from build123d import *

# Parameters (mm, degrees)
SKETCH1_R                                           = 18
BOSS_EXTRUDE1_DEPTH                                 = 7
CBORE_FOR_M4_HEX_SOCKET_HEAD_CAP_SCREW2_D           = 4.8
CBORE_FOR_M4_HEX_SOCKET_HEAD_CAP_SCREW2_DEPTH       = 10
CBORE_FOR_M4_HEX_SOCKET_HEAD_CAP_SCREW2_CBORE_D     = 8.2
CBORE_FOR_M4_HEX_SOCKET_HEAD_CAP_SCREW2_CBORE_DEPTH = 4.4
CBORE_FOR_M4_HEX_SOCKET_HEAD_CAP_SCREW2_TIP         = 1.442065486
F_3_0MM_DOWEL_HOLE1_D                               = 3
F_3_0MM_DOWEL_HOLE1_DEPTH                           = 10
F_3_0MM_DOWEL_HOLE1_TIP                             = 0.901290929
F_3_0MM_DOWEL_HOLE2_D                               = 3
F_3_0MM_DOWEL_HOLE2_DEPTH                           = 10
F_3_0MM_DOWEL_HOLE2_TIP                             = 0.901290929
SKETCH8_R                                           = 8
BOSS_EXTRUDE2_DEPTH                                 = 3
TAP_DRILL_FOR_M8_TAP1_D                             = 6.8


with BuildPart() as part:
    # Sketch1 → Boss-Extrude1 (new body)
    with BuildSketch(Plane(origin=(0, 0, 0), x_dir=(1, 0, 0), z_dir=(0, 1, 0))):
        with Locations(Location((0, 0, 0), (0, 0, 270))):
            Circle(SKETCH1_R)
    extrude(amount=BOSS_EXTRUDE1_DEPTH)

    # CBORE for M4 Hex Socket Head Cap Screw2
    with Locations(Plane(origin=(0, 7, 0), x_dir=(1, 0, 0), z_dir=(0, 1, 0))):
        with Locations((-12.124355653, 7), (0, 14), (12.124355653, 7), (12.124355653, -7), (0, -14), (-12.124355653, -7)):
            CounterBoreHole(CBORE_FOR_M4_HEX_SOCKET_HEAD_CAP_SCREW2_D / 2, CBORE_FOR_M4_HEX_SOCKET_HEAD_CAP_SCREW2_CBORE_D / 2, CBORE_FOR_M4_HEX_SOCKET_HEAD_CAP_SCREW2_CBORE_DEPTH, depth=CBORE_FOR_M4_HEX_SOCKET_HEAD_CAP_SCREW2_DEPTH)
            with Locations((0, 0, -(CBORE_FOR_M4_HEX_SOCKET_HEAD_CAP_SCREW2_DEPTH + CBORE_FOR_M4_HEX_SOCKET_HEAD_CAP_SCREW2_TIP / 2))):  # 118° drill point
                Cone(0, CBORE_FOR_M4_HEX_SOCKET_HEAD_CAP_SCREW2_D / 2, CBORE_FOR_M4_HEX_SOCKET_HEAD_CAP_SCREW2_TIP, mode=Mode.SUBTRACT)

    # Ø3.0mm Dowel Hole1
    with Locations(Plane(origin=(0, 7, 0), x_dir=(1, 0, 0), z_dir=(0, 1, 0))):
        with Locations((7, -12.124355653), (-14, 0), (7, 12.124355653)):
            Hole(F_3_0MM_DOWEL_HOLE1_D / 2, depth=F_3_0MM_DOWEL_HOLE1_DEPTH)
            with Locations((0, 0, -(F_3_0MM_DOWEL_HOLE1_DEPTH + F_3_0MM_DOWEL_HOLE1_TIP / 2))):  # 118° drill point
                Cone(0, F_3_0MM_DOWEL_HOLE1_D / 2, F_3_0MM_DOWEL_HOLE1_TIP, mode=Mode.SUBTRACT)

    # Ø3.0mm Dowel Hole2
    with Locations(Plane(origin=(0, 7, 0), x_dir=(1, 0, 0), z_dir=(0, 1, 0))):
        with Locations((-6.1, 10.565509926), (12.2, 0), (-6.1, -10.565509926)):
            Hole(F_3_0MM_DOWEL_HOLE2_D / 2, depth=F_3_0MM_DOWEL_HOLE2_DEPTH)
            with Locations((0, 0, -(F_3_0MM_DOWEL_HOLE2_DEPTH + F_3_0MM_DOWEL_HOLE2_TIP / 2))):  # 118° drill point
                Cone(0, F_3_0MM_DOWEL_HOLE2_D / 2, F_3_0MM_DOWEL_HOLE2_TIP, mode=Mode.SUBTRACT)

    # Sketch8 → Boss-Extrude2 (add)
    with BuildSketch(Plane(origin=(0, 7, 0), x_dir=(1, 0, 0), z_dir=(0, 1, 0))):
        with Locations(Location((0, 0, 0), (0, 0, 270))):
            Circle(SKETCH8_R)
    extrude(amount=BOSS_EXTRUDE2_DEPTH)

    # Tap Drill for M8 Tap1 (through all)
    with Locations(Plane(origin=(0, 10, 0), x_dir=(1, 0, 0), z_dir=(0, 1, 0))):
        with Locations((0, 0)):
            Hole(TAP_DRILL_FOR_M8_TAP1_D / 2)


solid = part.part
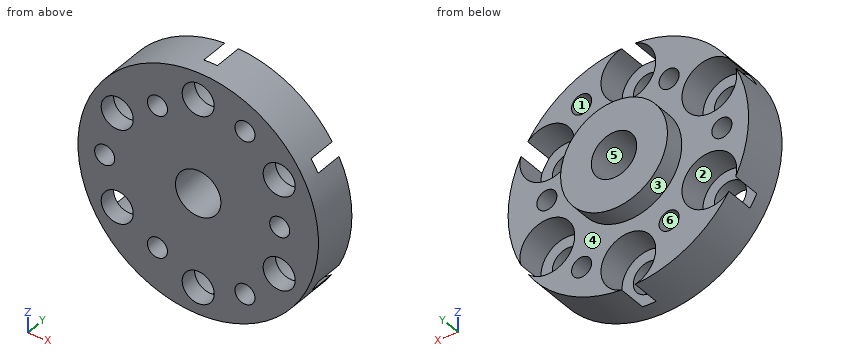
Build history of the part. All positions in model axes, mm. Face numbers are marked on the shaded views. A direction names the side the tool comes from. Coordinates: 2 decimals unless noted, no trailing zeros. Order: outer loops, then holes, each group sorted by start corner. A loop starts at its lowest first (then second) coordinate and runs counter-clockwise, first axis right, second up. Notation, with made-up numbers: (-26.5, 58.5) - (-13.5, 58.5) arc R18 cw to (-13.5, 70.5) - close; hole circle Ø9 at (64, 64.5). An arc over 180 degrees is marked (long way). Put each result on its own line as item: value.
1. Saw through at B-B (z = 0). Write the cut outline in (x, y).
Answer sheet:
outline: (-18, 0) - (-15.5, 0) - (-15.5, 7) - (-18, 7) - close; (-12.5, 0) - (-3.4, 0) - (-3.4, 10) - (-8, 10) - (-8, 7) - (-12.5, 7) - close; (3.4, 0) - (10.7, 0) - (10.7, 7) - (8, 7) - (8, 10) - (3.4, 10) - close; (13.7, 0) - (18, 0) - (18, 7) - (13.7, 7) - close
2. Tool access for the marked faces 1 and 2: list every direction of +Z, -Z, +X, -X, +Y, -Y with a clear straight run to the whole face (end or side of a thin tool).
Answer sheet:
face 1: +Y, -Y
face 2: +Y
3. Pull direction X, two halves, no side cores. Call the marked faces 3, 4, 5 and 6: pulls with the +X half, pulls with the -X half, needs draft (parallel to the pull), parting line crosses it, or undercut.
Answer sheet:
face 3: parting line crosses it
face 4: needs draft
face 5: undercut
face 6: undercut
4. Probe line 1 along Z through (x, y) = (0, 4.4); line 2 along Z through (x, y) = (-2, 4.5); line 3 along X through (y, z) = (6.25, 13.5). List the from-to ranges inside material, lowest first. Write a range as [from, to].
Answer sheet:
line 1: z = [-9.9, -3.4], [3.4, 9.9]
line 2: z = [-17.89, -17.58], [-10.42, -2.75], [2.75, 10.42], [17.58, 17.89]
line 3: x = [-11.91, -4.07], [4.07, 6.4], [7.6, 11.91]
5. Saw through at C-C (z = -15). Write the cut outline in (x, y), and give its area (3 significant figures).
Answer sheet:
outline: (-9.95, 0) - (-2.18, 0) - (-2.18, 2.6) - (-3.98, 2.6) - (-3.98, 7) - (-9.95, 7) - close; (2.18, 0) - (9.95, 0) - (9.95, 7) - (3.98, 7) - (3.98, 2.6) - (2.18, 2.6) - close
area: 93.0 mm^2
6. Drop flat-ended pins along their axis: P1, Ø5, axis at x = 0, z = 14, coming from the +Y side; P2, Ø4, axis at x = -14, y = 1.5, coming from the +Z side; P3, Ø6, axis at x = -14, y = 3, coming from the +Z side. Give the stop position or say it passes through.
Answer sheet:
P1: stops at y = 2.6
P2: stops at z = 13.42
P3: stops at z = 14.25
7. Saw through at A-A (x = 0). Write the cut outline in (y, z).
Answer sheet:
outline: (0, -18) - (2.6, -18) - (2.6, -16.4) - (0, -16.4) - close; (0, -11.6) - (2.6, -11.6) - (2.6, -9.9) - (7, -9.9) - (7, -8) - (10, -8) - (10, -3.4) - (0, -3.4) - close; (0, 3.4) - (10, 3.4) - (10, 8) - (7, 8) - (7, 9.9) - (2.6, 9.9) - (2.6, 11.6) - (0, 11.6) - close; (0, 16.4) - (2.6, 16.4) - (2.6, 18) - (0, 18) - close
8. Saw through at D-D (y = 5.25). Write the cut outline in (x, z), and give its area (3 significant figures).
Answer sheet:
outline: (-16.07, -8.1) arc R4.1 cw (long way) to (-15.05, -9.87) arc R18 ccw to (-1.02, -17.97) arc R4.1 cw (long way) to (1.02, -17.97) arc R18 ccw to (15.05, -9.87) arc R4.1 cw (long way) to (16.07, -8.1) arc R18 ccw to (16.07, 8.1) arc R4.1 cw (long way) to (15.05, 9.87) arc R18 ccw to (1.02, 17.97) arc R4.1 cw (long way) to (-1.02, 17.97) arc R18 ccw to (-15.05, 9.87) arc R4.1 cw (long way) to (-16.07, 8.1) arc R18 ccw to start; hole circle Ø3 at (-14, 0); hole circle Ø3 at (-6.1, -10.57); hole circle Ø3 at (-6.1, 10.57); hole circle Ø6.8 at (0, 0); hole circle Ø3 at (7, -12.12); hole circle Ø3 at (7, 12.12); hole circle Ø3 at (12.2, 0)
area: 623 mm^2
